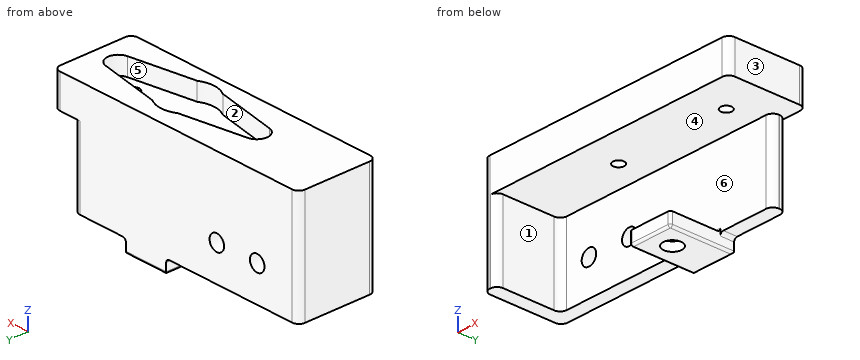
```python
from build123d import *

# Parameters (mm, degrees)
SKETCH1_W                       = 75.438
SKETCH1_H                       = 12.7
BOSS_EXTRUDE1_DEPTH             = 6.35
CUT_EXTRUDE1_DEPTH              = 4
BOSS_EXTRUDE2_REACH             = 40.773
SKETCH3_W                       = 75.438
SKETCH3_H                       = 19.05
SKETCH3_W_2                     = 69.088
SKETCH3_H_2                     = 12.7
BOSS_EXTRUDE2_DIRECTION_2_REACH = 40.773
SKETCH4_W                       = 75.438
SKETCH4_H                       = 25.4
BOSS_EXTRUDE4_DEPTH             = 3.175
SKETCH7_W                       = 14.859
SKETCH7_H                       = 15.875
CUT_EXTRUDE3_DEPTH              = 47.460828512
SKETCH8_W                       = 3.175
SKETCH8_H                       = 15.875
CUT_EXTRUDE4_DEPTH              = 65.214043371
BOSS_EXTRUDE5_DEPTH             = 3.175
SKETCH11_W                      = 57.404
SKETCH11_H                      = 12.7
CUT_EXTRUDE5_DEPTH              = 2
SKETCH12_R                      = 1.27
CUT_EXTRUDE6_DEPTH              = 45.400547136
SKETCH10_R                      = 1.8
CUT_EXTRUDE7_DEPTH              = 45.123864983
SKETCH13_W                      = 17.875
SKETCH13_H                      = 3.175
CUT_EXTRUDE8_DEPTH              = 5
SKETCH14_W                      = 10
SKETCH14_H                      = 14.655071008
BOSS_EXTRUDE6_DEPTH             = 3
SKETCH15_R                      = 2.1
CUT_EXTRUDE9_DEPTH              = 2
BOSS_EXTRUDE7_DEPTH             = 2
FILLET3_R                       = 0.5
FILLET4_R                       = 0.75
FILLET5_R                       = 0.75
FILLET6_R                       = 0.75
FILLET2_R                       = 1.5


with BuildPart() as part:
    # Sketch1 → Boss-Extrude1 (new body)
    with BuildSketch(Plane.XY):
        Rectangle(SKETCH1_W, SKETCH1_H)
    extrude(amount=BOSS_EXTRUDE1_DEPTH)

    # Sketch2 → Cut-Extrude1 (cut)
    with BuildSketch(Plane.XY.offset(6.35)):
        with BuildLine():
            Line((3.175, 5.129369479), (17.6006647, 2.498793645))
            ThreePointArc((17.6006647, 2.498793645), (19.685, 0), (17.6006647, -2.498793645))
            Line((17.6006647, -2.498793645), (3.175, -5.129369479))
            ThreePointArc((3.175, -5.129369479), (0, -6.0325), (-3.175, -5.129369479))
            Line((-3.175, -5.129369479), (-17.6006647, -2.498793645))
            ThreePointArc((-17.6006647, -2.498793645), (-19.685, 0), (-17.6006647, 2.498793645))
            Line((-17.6006647, 2.498793645), (-3.175, 5.129369479))
            ThreePointArc((-3.175, 5.129369479), (0, 6.0325), (3.175, 5.129369479))
        make_face()
    extrude(amount=-CUT_EXTRUDE1_DEPTH, mode=Mode.SUBTRACT)

    # Boss-Extrude2: up to this face of the body (flat: up to its plane)
    boss_extrude2_end = Plane(part.part.faces().sort_by_distance((0, 6.35, 3.175))[0])
    # Sketch3 → Boss-Extrude2 (add, up to the picked face)
    with BuildSketch(Plane(origin=(0, 0, 0), x_dir=(1, 0, 0), z_dir=(0, 1, 0)), mode=Mode.PRIVATE) as boss_extrude2_sk1:
        with Locations((0, 9.525)):
            Rectangle(SKETCH3_W, SKETCH3_H)
        with Locations((0, 9.525)):
            Rectangle(SKETCH3_W_2, SKETCH3_H_2, mode=Mode.SUBTRACT)
    boss_extrude2_tool1 = split(extrude(boss_extrude2_sk1.sketch, amount=BOSS_EXTRUDE2_REACH, mode=Mode.PRIVATE), bisect_by=boss_extrude2_end, keep=Keep.BOTH, mode=Mode.PRIVATE)
    add(boss_extrude2_tool1.solids().sort_by(Axis((0, 0, -0.778061), (0, 1, 0)))[0])

    # Boss-Extrude2 direction 2: up to this face of the body (flat: up to its plane)
    boss_extrude2_direction_2_end = Plane(part.part.faces().sort_by_distance((0, -6.35, 3.175))[0])
    # Sketch3 → Boss-Extrude2 direction 2 (add, up to the picked face)
    with BuildSketch(Plane(origin=(0, 0, 0), x_dir=(1, 0, 0), z_dir=(0, 1, 0)), mode=Mode.PRIVATE) as boss_extrude2_direction_2_sk1:
        with Locations((0, 9.525)):
            Rectangle(SKETCH3_W, SKETCH3_H)
        with Locations((0, 9.525)):
            Rectangle(SKETCH3_W_2, SKETCH3_H_2, mode=Mode.SUBTRACT)
    boss_extrude2_direction_2_tool1 = split(extrude(boss_extrude2_direction_2_sk1.sketch, amount=-BOSS_EXTRUDE2_DIRECTION_2_REACH, mode=Mode.PRIVATE), bisect_by=boss_extrude2_direction_2_end, keep=Keep.BOTH, mode=Mode.PRIVATE)
    add(boss_extrude2_direction_2_tool1.solids().sort_by(Axis((0, 0, -0.778061), (0, -1, 0)))[0])

    # Sketch4 → Boss-Extrude4 (add)
    with BuildSketch(Plane(origin=(0, 6.35, 0), x_dir=(1, 0, 0), z_dir=(0, 1, 0))):
        with Locations((0, 6.35)):
            Rectangle(SKETCH4_W, SKETCH4_H)
    extrude(amount=BOSS_EXTRUDE4_DEPTH)

    # Sketch7 → Cut-Extrude3 (cut, through all)
    with BuildSketch(Plane.XY.offset(6.35)):
        with Locations((30.2895, 1.5875)):
            Rectangle(SKETCH7_W, SKETCH7_H)
    extrude(amount=-CUT_EXTRUDE3_DEPTH, mode=Mode.SUBTRACT)

    # Sketch8 → Cut-Extrude4 (cut, through all)
    with BuildSketch(Plane(origin=(22.86, 0, 0), x_dir=(0, 0, -1), z_dir=(1, 0, 0))):
        with Locations((17.4625, 1.5875)):
            Rectangle(SKETCH8_W, SKETCH8_H)
    extrude(amount=-CUT_EXTRUDE4_DEPTH, mode=Mode.SUBTRACT)

    # Sketch9 → Boss-Extrude5 (add)
    with BuildSketch(Plane(origin=(0, 0, -15.875), x_dir=(-1, 0, 0), z_dir=(0, 0, -1))):
        Polygon((34.544, 6.35), (34.544, -6.35), (37.719, -6.35), (37.719, 9.525), (-22.86, 9.525), (-22.86, 6.35), align=None)
    extrude(amount=BOSS_EXTRUDE5_DEPTH)

    # Sketch11 → Cut-Extrude5 (cut)
    with BuildSketch(Plane(origin=(0, 0, -3.175), x_dir=(-1, 0, 0), z_dir=(0, 0, -1))):
        with Locations((5.842, 0)):
            Rectangle(SKETCH11_W, SKETCH11_H)
    extrude(amount=-CUT_EXTRUDE5_DEPTH, mode=Mode.SUBTRACT)

    # Sketch12 → Cut-Extrude6 (cut, through all)
    with BuildSketch(Plane.XY.offset(2.35)):
        with Locations((13.335, 0)):
            Circle(SKETCH12_R)
        with Locations(Location((-13.335, 0, 0), (0, 0, 180))):
            Circle(SKETCH12_R)
    extrude(amount=-CUT_EXTRUDE6_DEPTH, mode=Mode.SUBTRACT)

    # Sketch10 → Cut-Extrude7 (cut, through all)
    with BuildSketch(Plane.XZ.offset(-6.35)):
        with Locations(Location((-27.544, -11.1125, 0), (0, 0, 270))):
            Circle(SKETCH10_R)
        with Locations(Location((-17.544, -11.1125, 0), (0, 0, 270))):
            Circle(SKETCH10_R)
    extrude(amount=-CUT_EXTRUDE7_DEPTH, mode=Mode.SUBTRACT)

    # Sketch13 → Cut-Extrude8 (cut)
    with BuildSketch(Plane(origin=(22.86, 0, 0), x_dir=(0, 0, -1), z_dir=(1, 0, 0))):
        with Locations((10.1125, 7.9375)):
            Rectangle(SKETCH13_W, SKETCH13_H)
    extrude(amount=-CUT_EXTRUDE8_DEPTH, mode=Mode.SUBTRACT)

    # Sketch14 → Boss-Extrude6 (add)
    with BuildSketch(Plane(origin=(0, 0, -19.05), x_dir=(-1, 0, 0), z_dir=(0, 0, -1))):
        with Locations((0, 2.197464496)):
            Rectangle(SKETCH14_W, SKETCH14_H)
    extrude(amount=BOSS_EXTRUDE6_DEPTH)

    # Sketch15 → Cut-Extrude9 (cut)
    with BuildSketch(Plane(origin=(0, 0, -22.05), x_dir=(-1, 0, 0), z_dir=(0, 0, -1))):
        Circle(SKETCH15_R)
    extrude(amount=-CUT_EXTRUDE9_DEPTH, mode=Mode.SUBTRACT)

    # Sketch16 → Boss-Extrude7 (add)
    with BuildSketch(Plane.XZ.offset(6.35)):
        Polygon((-34.544, -19.05), (-34.544, -1.175), (22.86, -1.175), (22.86, 6.35), (-37.719, 6.35), (-37.719, -19.05), align=None)
    extrude(amount=BOSS_EXTRUDE7_DEPTH)

    # Fillet3
    fillet3_edges = [part.edges().sort_by_distance(p)[0] for p in [
        (-5, -5.130071008, -20.55),
        (5, -5.130071008, -20.55),
        (-5, 2.197464496, -22.05),
        (0, 9.525, -22.05),
        (5, 2.197464496, -22.05),
        (0, -5.130071008, -22.05),
    ]]
    fillet(fillet3_edges, radius=FILLET3_R)

    # Fillet4
    # the kernel refuses this fillet: 0.75 mm, written as the material it adds along each edge
    with BuildSketch(Plane(origin=(5, 9.525, -19.05), x_dir=(0, 0, -1), z_dir=(0, -1, 0))) as fillet4_piece_1:
        with BuildLine():
            CenterArc((FILLET4_R, FILLET4_R), FILLET4_R, 180, 90)
            Line((0, FILLET4_R), (0, 0))
            Line((0, 0), (FILLET4_R, 0))
        make_face()
    extrude(amount=3.175)

    # Fillet5
    # the kernel refuses this fillet: 0.75 mm, written as the material it adds along each edge
    with BuildSketch(Plane(origin=(-5, 6.35, -19.05), x_dir=(0, 0, -1), z_dir=(0, 1, 0))) as fillet5_piece_1:
        with BuildLine():
            CenterArc((FILLET5_R, FILLET5_R), FILLET5_R, 180, 90)
            Line((0, FILLET5_R), (0, 0))
            Line((0, 0), (FILLET5_R, 0))
        make_face()
    extrude(amount=3.175)

    # Fillet6
    fillet6_edges = [part.edges().sort_by_distance(p)[0] for p in [
        (0, 6.35, -19.05),
    ]]
    fillet(fillet6_edges, radius=FILLET6_R)

    # Fillet2
    fillet2_edges = [part.edges().sort_by_distance(p)[0] for p in [
        (22.86, 9.525, 2.5875),
        (17.86, 9.525, -10.1125),
        (17.86, 6.35, -10.1125),
        (-34.544, -8.35, -10.1125),
        (22.86, -8.35, 2.5875),
        (-37.719, -8.35, -6.35),
        (-34.544, 6.35, -10.1125),
        (-37.719, 9.525, -6.35),
    ]]
    fillet(fillet2_edges, radius=FILLET2_R)


solid = part.part
```
The model under review builds one solid part; all positions refer to its coordinate system, in mm. Face numbers are marked on the shaded views. A direction names the side the tool comes from. Give positions to 0.01 mm unless a question says otherwise; leave off trailing zeros. Write each loop counter-clockwise with the first axis right and the second up, starting at its lowest first coordinate (ties: lowest second). Pieces come first, ordered by that corner, then holes.
(1) Consider section A-A, the plane y = 0. Give the boundary of the cut face in (x, z) (3 decimals).
(2) To check wall thickness, follow L1, parallel to Z at x = 2, y = 5 (3 decimals); L2, parallel to Y at x = 12, z = -6 (3 decimals); L3, parallel to X at y = 2.5, z = -17.25. State the ranges of each line that lie inside material, in increasing order.
(3) For P1, Ø3, axis at x = -13.335, y = 0, coming from the -Z side (3 decimals); P2, Ø8, axis at x = 10, z = -16, coming from the -Y side; P3, Ø0.8, axis at x = -1.5, z = -21, coming from the -Y side; P4, Ø3, axis at x = -27.54, z = -11.11, coming from the -Y side, all flat-tipped, find the tip position at first contact; note any pin that passes through.
(4) Tool access review of the marked faces 1, 2 and 3: name each direction out of +Z, -Z, +X, -X, +Y, -Y from which nothing blocks a thin tool from reaching the whole face with its end or side.
(5) Consider section C-C, the plane y = -3.25. Give the boundary of the cut face in (x, z) (3 decimals), and give its area (3 significant figures).
(6) The part is to be moulded in two halves that separate along Y. For the marked faces 4, 5 and 6, say which applies: released by +Y, released by -Y, zero draft, split by the parting line, or undercut.
Returned:
1. outline: (-37.719, -19.05) - (-34.544, -19.05) - (-34.544, -1.175) - (-14.605, -1.175) - (-14.605, 2.35) - (-19.685, 2.35) - (-19.685, 6.35) - (-37.719, 6.35) - close; (-12.065, -1.175) - (12.065, -1.175) - (12.065, 2.35) - (-12.065, 2.35) - close; (-5, -21.55) arc R0.5 ccw to (-4.5, -22.05) - (-2.1, -22.05) - (-2.1, -20.05) - (2.1, -20.05) - (2.1, -22.05) - (4.5, -22.05) arc R0.5 ccw to (5, -21.55) - (5, -19.05) - (-5, -19.05) - close; (14.605, -1.175) - (22.86, -1.175) - (22.86, 6.35) - (19.685, 6.35) - (19.685, 2.35) - (14.605, 2.35) - close
2. L1: z = -22.05 to -19.05, -1.175 to 2.35
2. L2: y = 6.35 to 9.525
2. L3: x = -37.72 to -34.54
3. P1: stops at z = -1.175
3. P2: stops at y = 6.35
3. P3: stops at y = -5.13
3. P4: passes through
4. face 1: -Z, +X, -Y
4. face 2: +Z
4. face 3: +Z, -Z, +X, +Y, -Y
5. outline: (-37.719, -19.05) - (-34.544, -19.05) - (-34.544, -1.175) - (22.86, -1.175) - (22.86, 6.35) - (13.481, 6.35) - (13.481, 2.35) - (-13.481, 2.35) - (-13.481, 6.35) - (-37.719, 6.35) - close; (-5, -21.55) arc R0.5 ccw to (-4.5, -22.05) - (4.5, -22.05) arc R0.5 ccw to (5, -21.55) - (5, -19.05) - (-5, -19.05) - close
5. area: 435 mm2
6. face 4: zero draft
6. face 5: undercut
6. face 6: released by -Y
